The listing builds one solid part. Answer for the finished solid, in the listing's coordinates (mm). Coordinates: 2 decimals unless noted, no trailing zeros. Write each loop counter-clockwise with the first axis right and the second up, starting at its lowest first coordinate (ties: lowest second). Pieces come first, ordered by that corner, then holes.
(1) Straight lines are drawn through the part: line 1 (Z direction, x = 25.95, y = 0) (3 decimals); line 2 (Y direction, x = 24.8, z = 72) (3 decimals); line 3 (Z direction, x = 25.3, y = -0.75). For each, find the intervals that lie inside material, in ascending order.
(2) The part is cut by section A-A on z = 20. Determine the outline of the cut face in (x, y).
(3) Given P1, Ø4, axis at y = 0, z = 20, coming from the +X side; P2, Ø5, axis at y = 0.5, z = 17, coming from the -X side; P3, Ø0.8, axis at x = 25.5, y = -5, coming from the -Z side, each flat-ended and moving along its own axis, determine where each tip first touches the part or whether it passes through.
(4) The part is cut by section B-B on z = 64. Determine the outline of the cut face in (x, y) (3 decimals).
(5) The part is cut by section C-C on x = 26.6. Give the number of separate pieces and of enclosed holes in the cut face, plus the area to 3 significant figures.
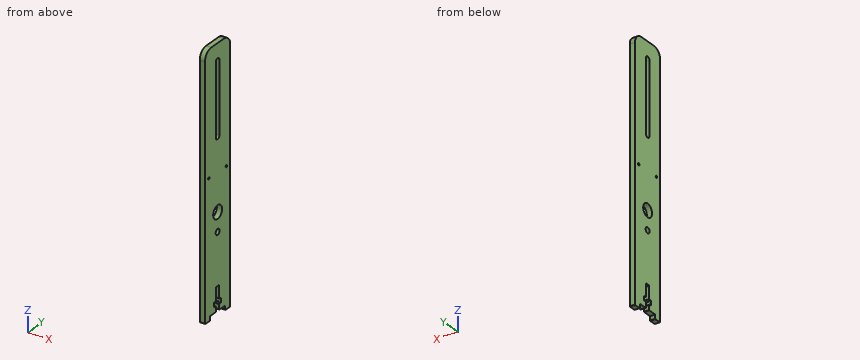
from build123d import *

# Parameters (mm, degrees)
SKETCH001_R             = 1.55
SKETCH001_R_2           = 0.6
PAD004_DEPTH            = 2.8
FILLET_R                = 0.4
FILLET001_R             = 5
SKETCH019_R             = 3.5
POCKET_DEPTH            = 2.801
BODY014_PLACEMENT_ANGLE = 180


with BuildPart() as part:
    # Sketch001 (on DatumPlane) → Pad004 (new body)
    with BuildSketch(Plane(origin=(-24.3, 0, 0), x_dir=(0, -1, 0), z_dir=(-1, 0, 0))):
        Polygon((-10, 85), (10, 85), (10, -52), (6, -52), (6, -49.7), (1.25, -49.7), (1.25, -46.7), (2.75, -46.7), (2.75, -44.2), (1.25, -44.2), (1.25, -37.2), (-1.25, -37.2), (-1.25, -44.2), (-2.75, -44.2), (-2.75, -46.7), (-1.25, -46.7), (-1.25, -49.7), (-6, -49.7), (-6, -52), (-10, -52), align=None)
        with Locations((0, -10)):
            Circle(SKETCH001_R, mode=Mode.SUBTRACT)
        with Locations((-7, 20)):
            Circle(SKETCH001_R_2, mode=Mode.SUBTRACT)
        with Locations((7, 20)):
            Circle(SKETCH001_R_2, mode=Mode.SUBTRACT)
        with BuildLine():
            ThreePointArc((1.425, 76), (0, 77.425), (-1.425, 76))
            Line((-1.425, 76), (-1.425, 38))
            ThreePointArc((-1.425, 38), (0, 36.575), (1.425, 38))
            Line((1.425, 38), (1.425, 76))
        make_face(mode=Mode.SUBTRACT)
    extrude(amount=PAD004_DEPTH)

    # Fillet
    fillet_edges = [part.edges().sort_by_distance(p)[0] for p in [
        (-25.7, 10, -52),
        (-25.7, 6, -52),
        (-25.7, -10, -52),
        (-25.7, -6, -52),
        (-25.7, 1.25, -49.7),
        (-25.7, -1.25, -49.7),
        (-25.7, 1.25, -37.2),
        (-25.7, -1.25, -37.2),
        (-25.7, 1.25, -46.7),
        (-25.7, -1.25, -46.7),
        (-25.7, 1.25, -44.2),
        (-25.7, -1.25, -44.2),
        (-25.7, -2.75, -46.7),
        (-25.7, 2.75, -46.7),
        (-25.7, 2.75, -44.2),
        (-25.7, -2.75, -44.2),
    ]]
    fillet(fillet_edges, radius=FILLET_R)

    # Fillet001
    fillet001_edges = [part.edges().sort_by_distance(p)[0] for p in [
        (-25.7, 10, 85),
        (-25.7, -10, 85),
    ]]
    fillet(fillet001_edges, radius=FILLET001_R)

    # Sketch019 (on Face47 of Fillet001) → Pocket (cut, through all)
    with BuildSketch(Plane(origin=(-27.1, 0, 0), x_dir=(0, -1, 0), z_dir=(-1, 0, 0))):
        Circle(SKETCH019_R)
    extrude(amount=-POCKET_DEPTH, mode=Mode.SUBTRACT)


with BuildPart() as part_1:
    # Body014 placement: moved
    add(part.part.moved(Location((0, 0, 20))).rotate(Axis((0, 0, 20), (0, 0, 1)), BODY014_PLACEMENT_ANGLE))


solid = part_1.part
Model answer:
1. line 1: z = -17.2 to 8.45, 11.55 to 16.5, 23.5 to 56.575, 97.425 to 105
1. line 2: y = -10 to -1.425, 1.425 to 10
1. line 3: z = -17.2 to 8.64, 11.36 to 16.58, 23.42 to 56.79, 97.21 to 105
2. outline: (24.3, -10) - (27.1, -10) - (27.1, -3.5) - (24.3, -3.5) - close; (24.3, 3.5) - (27.1, 3.5) - (27.1, 10) - (24.3, 10) - close
3. P1: passes through
3. P2: stops at x = 24.3
3. P3: stops at z = -29.7
4. outline: (24.3, -10) - (27.1, -10) - (27.1, -1.425) - (24.3, -1.425) - close; (24.3, 1.425) - (27.1, 1.425) - (27.1, 10) - (24.3, 10) - close
5. separate pieces: 1
5. enclosed holes: 5
5. area: 2,500 mm2
